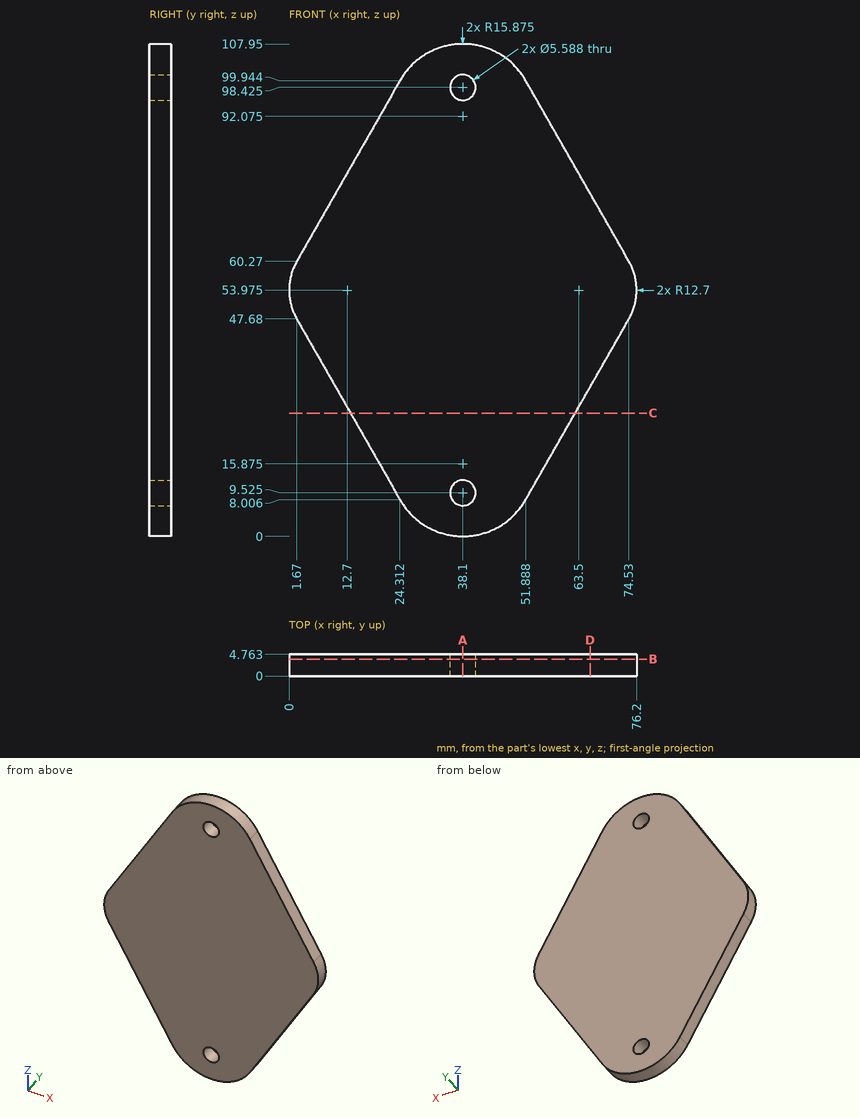
Print and shaded views of the part. All mm, measured from the part's lowest x, y and z. Give positions to 0.01 mm unless a question says otherwise; leave off trailing zeros. Write each loop counter-clockwise with the first axis right and the second up, starting at its lowest first coordinate (ties: lowest second). Pieces come first, ordered by that corner, then holes. Notation, with made-up numbers: (31.5, 52) -> (67.5, 52) arc R4 cw to (67.5, 58) -> close; hole circle Ø1 at (10.5, -8). An arc over 180 degrees is marked (long way). Use CSV: the item, a comma, the result in double quotes. Start each with the question number.
1) Drill centre lines: L1, parallel to Z at x = 38.1, y = 2.7; L2, parallel to X at y = 0.7, z = 11.5 (1 decimal); L3, parallel to Z at x = 41, y = 0.65. Where is each one in solid material? Low to high.
2) Cut at A-A on x = 38.1. List the corners of the cut face in (y, z).
3) Cut at B-B on y = 3.7. Count the separate pieces of the cut face and the enclosed holes in it.
4) Cut at C-C on z = 27. List the corners of the cut face in (x, y).
5) Cut at D-D on x = 66. List the corners of the cut face in (y, z), plus the area to 3 significant figures.
6) Pin check, flat tips, straight feed: P1, Ø1, axis at y = 3, z = 33.5, coming from the -X side; P2, Ø2, axis at y = 1.5, z = 23, coming from the -X side (1 decimal); P3, Ø2, axis at y = 4, z = 41, coming from the +X side. Stop position of each tip, or through.
Final values:
1,L1,"z = 0 to 6.73, 12.32 to 95.63, 101.22 to 107.95"
1,L2,"x = 22.3 to 36.1, 40.1 to 53.9"
1,L3,"z = 0.27 to 107.68"
2,outline,"(0, 0) -> (4.76, 0) -> (4.76, 6.73) -> (0, 6.73) -> close; (0, 12.32) -> (4.76, 12.32) -> (4.76, 95.63) -> (0, 95.63) -> close; (0, 101.22) -> (4.76, 101.22) -> (4.76, 107.95) -> (0, 107.95) -> close"
3,separate pieces,"1"
3,enclosed holes,"2"
4,outline,"(13.47, 0) -> (62.73, 0) -> (62.73, 4.76) -> (13.47, 4.76) -> close"
5,outline,"(0, 32.73) -> (4.76, 32.73) -> (4.76, 75.22) -> (0, 75.22) -> close"
5,area,"202 mm2"
6,P1,"stops at x = 9.48"
6,P2,"stops at x = 15.2"
6,P3,"stops at x = 71.29"
